CAD build for the part. Positions are in the model's coordinates, mm. A direction names the side the tool comes from. Round coordinates to 2 decimals unless told otherwise and drop trailing zeros. Loops run counter-clockwise (first coordinate to the right, second up) from the corner with the lowest first, then second, coordinate; pieces in that order, holes last. Notation, with made-up numbers: M -2,23 L 37,23 A38 cw 37,62 Z; hole C -1,74.5 d1. An arc over 180 degrees is marked long. Put each result on its own line as item: value. Start each with the question number.
from build123d import *

# Parameters (mm, degrees)
F0_R     = 55
F0_R_2   = 51
F0_R_3   = 46
F1_DEPTH = 7
F2_DEPTH = 500
F3_DEPTH = 100
F4_R     = 10


with BuildPart() as f1:
    # F0 (on Top) → F1 (new body)
    with BuildSketch(Plane.XY):
        Circle(F0_R)
        Circle(F0_R_2, mode=Mode.SUBTRACT)
        Circle(F0_R_2)
        Circle(F0_R_3, mode=Mode.SUBTRACT)
        Circle(F0_R_3)
    extrude(amount=F1_DEPTH)

    # F0 (on Top) → F2 (join)
    with BuildSketch(Plane.XY):
        Circle(F0_R_2)
        Circle(F0_R_3, mode=Mode.SUBTRACT)
    extrude(amount=-F2_DEPTH)

    # F0 (on Top) → F3 (join)
    with BuildSketch(Plane.XY):
        Circle(F0_R)
        Circle(F0_R_2, mode=Mode.SUBTRACT)
    extrude(amount=-F3_DEPTH)

    # F4
    f4_edges = [f1.edges().sort_by_distance(p)[0] for p in [
        (-55, 0, 7),
    ]]
    fillet(f4_edges, radius=F4_R)


solid = f1.part
(1) Cut at D-D on z = -216. List the corners of the cut face in (x, y).
(2) Cut at C-C on z = -67. List the corners of the cut face in (x, y).
(3) Drill centre lines: line 1 along Y through (x, z) = (0, -359.5); line 2 along X through (y, z) = (1, -428.5); line 3 along X through (y, z) = (36.5, -51). Where is each one in solid material? Low to high.
(4) Mould opens along Y. For faces 1 (the cylindrical face through (-11.923, -53.692, -50.821)), 2 (the cylindrical face through (-5.99, 45.61, -246.5)), 3 (the flat face through (-1, 1, 7)) say: +Y half, -Y half, draft (parallel to the pull), parting line (faces both ways), or undercut.
(5) Tool access for faces 4 (the flat face through (-8, 46, -500)), 5 (the cylindrical face through (-11.056, -49.787, -297.2)): list every direction of +Z, -Z, +X, -X, +Y, -Y with a clear straight run to the whole face (end or side of a thin tool).
(6) Flat gauge pins, fed straight in: pin 1 Ø12 at (y, z) = (31, -104.5) entering from +X; pin 2 Ø6 at (x, y) = (-41.5, 39.5) entering from -Z; pin 3 Ø3 at (x, z) = (-39, -221.5) entering from -Y. Where does each tip first touch, or does it go through?
(7) Cut at A-A on x = 0. List the corners of the cut face in (y, z).
Taken from the geometry:
1. outline: C 0,0 d102; hole C 0,0 d92
2. outline: C 0,0 d110; hole C 0,0 d92
3. line 1: -51 to -46, 46 to 51
3. line 2: -50.99 to -45.99, 45.99 to 50.99
3. line 3: -41.14 to -28, 28 to 41.14
4. face 1: parting line
4. face 2: undercut
4. face 3: draft
5. face 4: -Z, +X, -X, +Y, -Y
5. face 5: -Z
6. pin 1: x = 47.9
6. pin 2: z = -100
6. pin 3: y = -34.57
7. outline: M -55,-100 L -51,-100 L -51,-500 L -46,-500 L -46,0 L 46,0 L 46,-500 L 51,-500 L 51,-100 L 55,-100 L 55,-3 A10 ccw 45,7 L -45,7 A10 ccw -55,-3 Z
